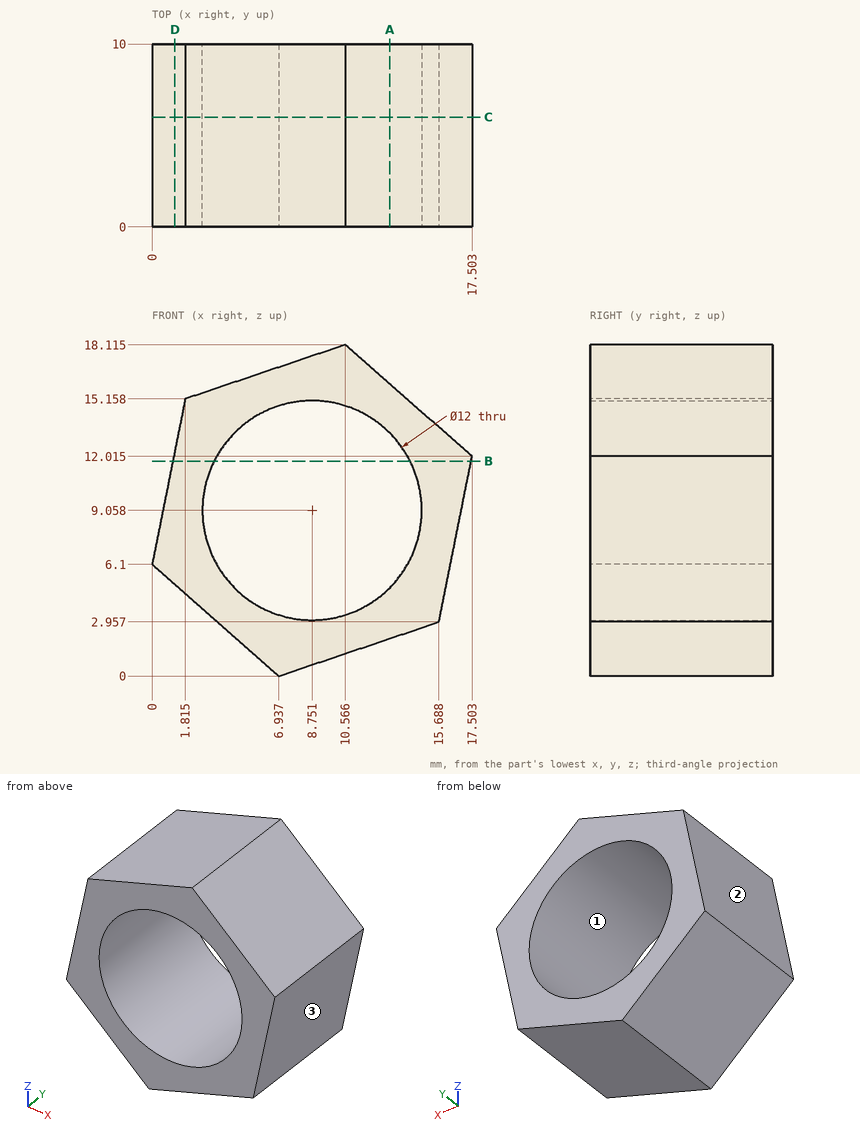
Study the drawing (mm; zero at the part's minimum x, y, z) and answer. Give positions to 0.01 mm unless a question says otherwise; leave off trailing zeros. Loops run counter-clockwise (first coordinate to the right, second up) from the corner with the lowest first, then second, coordinate; pieces in that order, holes last. Notation, with made-up numbers: (43.5, -22.5) - (73.5, -22.5) arc R18 ccw to (73.5, 2.5) - close; hole circle Ø4 at (15.25, 74.5). An arc over 180 degrees is marked (long way). Use CSV: the item, a comma, the result in double quotes. Start each with the question number.
(1) Find the intervals of material crossed by L1, parallel to Z at x = 11.5, y = 1.5 (1 decimal); L2, parallel to Z at x = 10.5, y = 8.5 (1 decimal); L3, parallel to X at y = 8.5, z = 13 (1 decimal), in increasing order.
(2) Find section B-B, the plane z = 11.75. Determine the outline of the cut face in (x, y).
(3) Find section A-A, the plane x = 13. Determine the outline of the cut face in (y, z) (1 decimal).
(4) Determine the mould class of the marked faces 1, 2 and 3 for opening direction Z: released by +Z, released by -Z, zero draft, split by the parting line, or undercut.
(5) Find section C-C, the plane y = 6. Determine the outline of the cut face in (x, z) (1 decimal).
(6) Each of these flat-tipped pins is pushed along its axis until it touches: pin 1 (3 mm diameter, centred on y = 7, z = 7, fed in from +X); pin 2 (4 mm diameter, centred on x = 2.5, z = 12, fed in from -Y); pin 3 (5 mm diameter, centred on y = 1.5, z = 9, fed in from +X); pin 4 (3 mm diameter, centred on x = 3.5, y = 2.5, fed in from -Z). Where does it stop, or does it pass through?
(7) Find section D-D, the plane x = 1.25. Determine the outline of the cut face in (y, z), plus the area to 3 significant figures.
Results found:
1,L1,"1.5 to 3.7, 14.4 to 17.3"
1,L2,"1.2 to 3.3, 14.8 to 18.1"
1,L3,"1.4 to 4.2, 13.3 to 16.4"
2,outline,"(1.13, 0) - (3.39, 0) - (3.39, 10) - (1.13, 10) - close; (14.11, 0) - (17.45, 0) - (17.45, 10) - (14.11, 10) - close"
3,outline,"(0, 2) - (10, 2) - (10, 4.8) - (0, 4.8) - close; (0, 13.3) - (10, 13.3) - (10, 16) - (0, 16) - close"
4,face 1,"undercut"
4,face 2,"released by +Z"
4,face 3,"released by -Z"
5,outline,"(0, 6.1) - (6.9, 0) - (15.7, 3) - (17.5, 12) - (10.6, 18.1) - (1.8, 15.2) - close; hole circle Ø12 at (8.8, 9.1)"
6,pin 1,"x = 16.8"
6,pin 2,"y = 0"
6,pin 3,"x = 17.4"
6,pin 4,"z = 1.7"
7,outline,"(0, 5) - (10, 5) - (10, 12.34) - (0, 12.34) - close"
7,area,"73.4 mm^2"
